from build123d import *

# Parameters (mm, degrees)
SKETCH1_R                       = 26
SKETCH1_R_2                     = 21.25
BOSS_EXTRUDE1_DEPTH             = 9
BOSS_EXTRUDE2_START             = 2
SKETCH2_R                       = 26
SKETCH2_R_2                     = 18
BOSS_EXTRUDE2_DEPTH             = 2
BOSS_EXTRUDE3_REACH             = 40.38
SKETCH3_W                       = 10.75
SKETCH3_H                       = 28
BOSS_EXTRUDE3_DIRECTION_2_DEPTH = 18
SKETCH4_R                       = 11.15
CUT_EXTRUDE1_DEPTH              = 7
CUT_EXTRUDE2_START              = -7
SKETCH5_R                       = 11.15
CUT_EXTRUDE2_DEPTH              = 7
SKETCH6_R                       = 8
CUT_EXTRUDE3_DEPTH              = 69.220231603
FILLET2_R                       = 14
FILLET3_R                       = 10
FILLET4_R                       = 1


with BuildPart() as part:
    # Sketch1 → Boss-Extrude1 (new body)
    with BuildSketch(Plane(origin=(0, 0, 0), x_dir=(1, 0, 0), z_dir=(0, 1, 0))):
        with Locations(Location((0, 0, 0), (0, 0, 270))):
            Circle(SKETCH1_R)
        with Locations(Location((0, 0, 0), (0, 0, 270))):
            Circle(SKETCH1_R_2, mode=Mode.SUBTRACT)
    extrude(amount=BOSS_EXTRUDE1_DEPTH)

    # Sketch2 → Boss-Extrude2 (add)
    with BuildSketch(Plane.XZ.offset(BOSS_EXTRUDE2_START)):
        with Locations(Location((0, 0, 0), (0, 0, 270))):
            Circle(SKETCH2_R)
        with Locations(Location((0, 0, 0), (0, 0, 270))):
            Circle(SKETCH2_R_2, mode=Mode.SUBTRACT)
    extrude(amount=-BOSS_EXTRUDE2_DEPTH)

    # Boss-Extrude3: up to this face of the body (flat: up to its plane)
    boss_extrude3_end = Plane(part.part.faces().sort_by_distance((0, -2, 25.264608948))[0])
    # Sketch3 → Boss-Extrude3 (add, up to the picked face)
    with BuildSketch(Plane(origin=(0, 9, 0), x_dir=(1, 0, 0), z_dir=(0, 1, 0)), mode=Mode.PRIVATE) as boss_extrude3_sk1:
        with Locations((26.625, 0)):
            Rectangle(SKETCH3_W, SKETCH3_H)
    boss_extrude3_tool1 = split(extrude(boss_extrude3_sk1.sketch, amount=-BOSS_EXTRUDE3_REACH, mode=Mode.PRIVATE), bisect_by=boss_extrude3_end, keep=Keep.BOTH, mode=Mode.PRIVATE)
    # Sketch3 → Boss-Extrude3 (add, up to the picked face)
    with BuildSketch(Plane(origin=(0, 9, 0), x_dir=(1, 0, 0), z_dir=(0, 1, 0)), mode=Mode.PRIVATE) as boss_extrude3_sk2:
        with Locations((-26.625, 0)):
            Rectangle(SKETCH3_W, SKETCH3_H)
    boss_extrude3_tool2 = split(extrude(boss_extrude3_sk2.sketch, amount=-BOSS_EXTRUDE3_REACH, mode=Mode.PRIVATE), bisect_by=boss_extrude3_end, keep=Keep.BOTH, mode=Mode.PRIVATE)
    add(boss_extrude3_tool1.solids().sort_by(Axis((26.625, 9, 0), (0, -1, 0)))[0])
    add(boss_extrude3_tool2.solids().sort_by(Axis((-26.625, 9, 0), (0, -1, 0)))[0])

    # Sketch3 → Boss-Extrude3 direction 2 (add)
    with BuildSketch(Plane(origin=(0, 9, 0), x_dir=(1, 0, 0), z_dir=(0, 1, 0))):
        with Locations((26.625, 0)):
            Rectangle(SKETCH3_W, SKETCH3_H)
        with Locations((-26.625, 0)):
            Rectangle(SKETCH3_W, SKETCH3_H)
    extrude(amount=BOSS_EXTRUDE3_DIRECTION_2_DEPTH)

    # Sketch4 → Cut-Extrude1 (cut)
    with BuildSketch(Plane(origin=(32, 0, 0), x_dir=(0, 0, -1), z_dir=(1, 0, 0))):
        with Locations((0, 13)):
            Circle(SKETCH4_R)
    extrude(amount=-CUT_EXTRUDE1_DEPTH, mode=Mode.SUBTRACT)

    # Sketch5 → Cut-Extrude2 (cut)
    with BuildSketch(Plane.ZY.offset(32).offset(CUT_EXTRUDE2_START)):
        with Locations(Location((0, 13, 0), (0, 0, 180))):
            Circle(SKETCH5_R)
    extrude(amount=CUT_EXTRUDE2_DEPTH, mode=Mode.SUBTRACT)

    # Sketch6 → Cut-Extrude3 (cut, through all)
    with BuildSketch(Plane(origin=(25, 0, 0), x_dir=(0, 0, -1), z_dir=(1, 0, 0))):
        with Locations(Location((0, 13, 0), (0, 0, 330))):
            Circle(SKETCH6_R)
    extrude(amount=-CUT_EXTRUDE3_DEPTH, mode=Mode.SUBTRACT)

    # Fillet2
    fillet2_edges = [part.edges().sort_by_distance(p)[0] for p in [
        (-26.625, 27, 14),
        (-26.625, 27, -14),
        (26.625, 27, -14),
        (26.625, 27, 14),
    ]]
    fillet(fillet2_edges, radius=FILLET2_R - 0.0001)  # a hair under: the kernel refuses the full size

    # Fillet3
    fillet3_edges = [part.edges().sort_by_distance(p)[0] for p in [
        (-21.9089023, 3.5, -14),
        (-21.9089023, 3.5, 14),
        (21.9089023, 3.5, -14),
        (21.9089023, 3.5, 14),
    ]]
    fillet(fillet3_edges, radius=FILLET3_R)

    # Fillet4
    fillet4_edges = [part.edges().sort_by_distance(p)[0] for p in [
        (-32, 5.50005, 14),
        (-32, 5.50005, -14),
        (-32, 22.899524226, -9.899524226),
        (-32, 22.899524226, 9.899524226),
        (32, 5.50005, -14),
        (32, 5.50005, 14),
        (32, 22.899524226, 9.899524226),
        (32, 22.899524226, -9.899524226),
    ]]
    fillet(fillet4_edges, radius=FILLET4_R)


solid = part.part
Model file for the job. Use its own axes, mm. A direction names the side the tool comes from. Coordinates: 2 decimals unless noted, no trailing zeros. Order: outer loops, then holes, each group sorted by start corner. A loop starts at its lowest first (then second) coordinate and runs counter-clockwise, first axis right, second up. Notation, with made-up numbers: (86.5, 17.5) -> (90.5, 17.5) arc R16 ccw to (90.5, 34.5) -> close; hole circle Ø10 at (-15.5, 54.25). An arc over 180 degrees is marked (long way). Return JSON: item names as keys, results as strings. Group by question number.
Item 1: Saw through at D-D on z = 15.5. Write the cut outline in (x, y).
Item 2: Saw through at B-B on y = 1. Write the cut outline in (x, z).
Item 3: Tool access for faces 5 (the flat face through (-28, 7, 14)), 6 (the cylindrical face through (28.5, 22.4, -6)), 7 (the flat face through (-28, 7, -14)): list every direction of +Z, -Z, +X, -X, +Y, -Y with a clear straight run to the whole face (end or side of a thin tool).
Item 4: Pull direction X, two halves, no side cores. Call faces 1 (the flat face through (15, -2, 12)), 2 (the flat face through (-32, 2, 6)), 3 (the flat face through (21.25, 22, 0)), 4 (the cylindrical face through (22.8, 3.42, -14.85)): pulls with the +X half, pulls with the -X half, needs draft (parallel to the pull), parting line crosses it, or undercut.
Item 5: Flat gauge pins, fed straight in: P1, Ø11, axis at y = 13, z = -3, coming from the -X side; P2, Ø4, axis at x = -5.5, z = -17, coming from the +Y side; P3, Ø10.5, axis at x = 28.5, y = 2.5, coming from the +Z side. Where does each tip first touch, or does it go through?
Item 6: Wall check: line 1 along Z through (x, y) = (0, 4.75); line 2 along Z through (x, y) = (22.85, 13); line 3 along X through (y, z) = (14.25, 8). Give the ranges that are in metal, low to high. Write a range as [from, to].
Item 7: Saw through at C-C on x = 0. Write the cut outline in (y, z), then the cut area to 4 significant figures.
Values found:
{
 "1": {"outline": "(-21.56, -2) -> (-9.15, -2) -> (-9.15, 0) -> (-14.54, 0) -> (-14.54, 9) -> (-21.56, 9) -> close; (9.15, -2) -> (21.56, -2) -> (21.56, 9) -> (14.54, 9) -> (14.54, 0) -> (9.15, 0) -> close"},
 "2": {"outline": "(-32, -13) arc R1 ccw to (-31, -14) -> (-26.83, -14) arc R10 cw to (-19.38, -17.33) arc R26 ccw to (19.38, -17.33) arc R10 cw to (26.83, -14) -> (31, -14) arc R1 ccw to (32, -13) -> (32, 13) arc R1 ccw to (31, 14) -> (26.83, 14) arc R10 cw to (19.38, 17.33) arc R26 ccw to (-19.38, 17.33) arc R10 cw to (-26.83, 14) -> (-31, 14) arc R1 ccw to (-32, 13) -> close; hole circle Ø42.5 at (0, 0)"},
 "3": {"face 5": "+Z, -X, +Y", "face 6": "+X", "face 7": "-Z, -X, +Y"},
 "4": {"face 1": "needs draft", "face 2": "pulls with the -X half", "face 3": "undercut", "face 4": "pulls with the +X half"},
 "5": {"P1": "stops at x = -25", "P2": "stops at y = 0", "P3": "stops at z = 14.66"},
 "6": {"line 1": "z = [-26, -21.25], [21.25, 26]", "line 2": "z = [-14, -8], [8, 14]", "line 3": "x = [-25, -21.25], [21.25, 25]"},
 "7": {"outline": "(-2, -26) -> (9, -26) -> (9, -21.25) -> (0, -21.25) -> (0, -18) -> (-2, -18) -> close; (-2, 18) -> (0, 18) -> (0, 21.25) -> (9, 21.25) -> (9, 26) -> (-2, 26) -> close", "area": "117.5 mm2"}
}
